Autodesk Fusion 360 part; units mm, degrees
sketch "Sketch2" plane through (0, 0, 0) normal (0, 0, 1) x (1, 0, 0)
  line L0 (0, 0) -> (2, 0)
  line L1 (2, 0) -> (2, 10)
  line L2 (2, 10) -> (0, 10)
  line L3 (0, 10) -> (0, 0)
  line L4 (0, 10) -> (2, 10)
  line L5 (2, 10) -> (2, 12)
  line L6 (2, 12) -> (0, 12)
  line L7 (0, 12) -> (0, 10)
  line L8 (0, 10) -> (-5, 10)
  line L9 (-5, 10) -> (-5, 12)
  line L10 (-5, 12) -> (0, 12)
  line L11 (0, 12) -> (0, 10)
  line L12 (-5, 10) -> (-7, 10)
  line L13 (-7, 10) -> (-7, 12)
  line L14 (-7, 12) -> (-5, 12)
  line L15 (-5, 12) -> (-5, 10)
  line L16 (-7, 10) -> (-5, 10)
  line L17 (-5, 10) -> (-5, -14)
  line L18 (-5, -14) -> (-7, -14)
  line L19 (-7, -14) -> (-7, 10)
  line L20 (-7, -14) -> (-5, -14)
  line L21 (-5, -14) -> (-5, -16)
  line L22 (-5, -16) -> (-7, -16)
  line L23 (-7, -16) -> (-7, -14)
  line L24 (-7, -16) -> (-30, -16)
  line L25 (-30, -16) -> (-30, -14)
  line L26 (-30, -14) -> (-7, -14)
  line L27 (-7, -14) -> (-7, -16)
  line L28 (-30, -16) -> (-32, -16)
  line L29 (-32, -16) -> (-32, -14)
  line L30 (-32, -14) -> (-30, -14)
  line L31 (-30, -14) -> (-30, -16)
  line L32 (-32, -14) -> (-30, -14)
  line L33 (-30, -14) -> (-30, 10)
  line L34 (-30, 10) -> (-32, 10)
  line L35 (-32, 10) -> (-32, -14)
  dimension "d3" = 2
  dimension "d4" = 10
  dimension "d5" = 2
  dimension "d6" = 2
  dimension "d7" = 5
  dimension "d8" = 2
  dimension "d9" = 2
  dimension "d10" = 2
  dimension "d11" = 24
  dimension "d12" = 2
  dimension "d13" = 23
  dimension "d14" = 2
  dimension "d15" = 2
  dimension "d16" = 2
  dimension "d17" = 2
  dimension "d18" = 24
extrude "Extrude1" add sketch "Sketch2" along normal blind 36
sketch "Sketch3" plane through (0, -16, 0) normal (0, -1, 0) x (1, 0, 0)
  line L0 (-32, 0) -> (-5, 0)
  line L1 (-5, 0) -> (-5, 36)
  line L2 (-5, 36) -> (-32, 36)
  line L3 (-32, 36) -> (-32, 0)
  line L4 (-5, 18) -> (-7, 18) construction
  line L5 (-7, 18) -> (-10.5, 18) construction
  line L6 (-14, 12) -> (-7, 12)
  line L7 (-7, 12) -> (-7, 24)
  line L8 (-7, 24) -> (-14, 24)
  line L9 (-14, 24) -> (-14, 12)
  line L10 (-14, 12) -> (-7, 24) construction
  line L11 (-7, 12) -> (-14, 24) construction
  point P0 (-7, 18)
  point P1 (-10.5, 18)
  dimension "d23" = 2
  dimension "d28" = 3.5
  dimension "d29" = 7
  dimension "d30" = 12
extrude "Extrude3" cut sketch "Sketch3" against normal blind 3 contours L6 L7 L8 L9
fillet "Fillet1" radius 0.5 8 edges at (0, 0, 18) (2, 0, 18) (-5, -16, 18) (-32, -16, 18) (2, 12, 18) (-7, 12, 18) (-30, 10, 18) (-32, 10, 18)
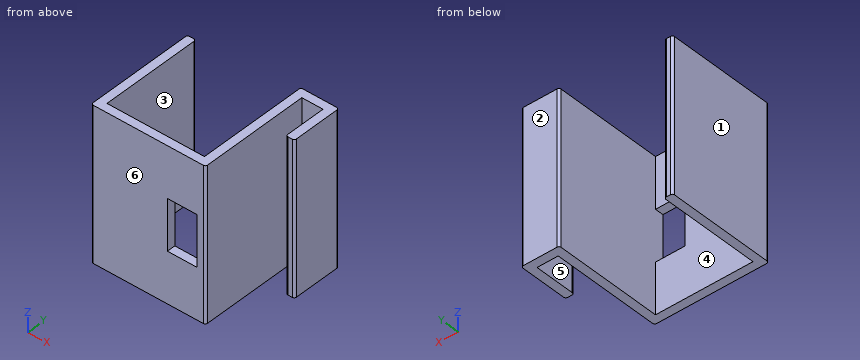
Verification items for the finished model (mm, model axes). Face numbers are marked on the shaded views. A direction names the side the tool comes from. Give positions to 0.01 mm unless a question says otherwise; leave off trailing zeros. Loops run counter-clockwise (first coordinate to the right, second up) from the corner with the lowest first, then second, coordinate; pieces in that order, holes last.
1. Mould release check, pull along X, two halves, no side actions. Record for the marked faces 1, 2 and 3: released by +X, released by -X, zero draft, split by the parting line, or undercut.
2. Set-up check for the marked faces 4, 5 and 6: record each of +Z, -Z, +X, -X, +Y, -Y from which the full face is reachable in a straight line by a thin tool's end or side.
3. Section check D-D, the plane x = -12.5. Enter the section's corners in (y, z), then the cut area to 3 significant figures.
4. Section check B-B, the plane y = -8.25. Enter the section's corners in (x, z), then the cut area to 3 significant figures.
5. Thickness scan on line 1 (X direction, y = 4.75, z = 20.5); line 2 (X direction, y = -8, z = 30.5); line 3 (X direction, y = -14.5, z = 14). Record the ranges inside material, lowest first.
6. Section check A-A, the plane y = 9. Enter the section's corners in (x, z).
7. Go/stop test with flat-tipped pins: pin 1 Ø1.1 at (x, z) = (1, 12.5) entering from -Y; pin 2 Ø0.6 at (y, z) = (-15, 20) entering from +X; pin 3 Ø5 at (x, z) = (-18, 23) entering from +Y; pin 4 Ø6 at (x, y) = (-19, -10) entering from +Z. Record where each tip stops, or that it passes through.
8. Section check C-C, the plane z = 13. Enter the section's corners in (x, y).
Geometry says:
1. face 1: released by -X
1. face 2: zero draft
1. face 3: undercut
2. face 4: +Z, -Z, +Y
2. face 5: +Z, -Z, -Y
2. face 6: +Z, -Z, +X, -X, -Y
3. outline: (-16, 0) - (-14, 0) - (-14, 12) - (-16, 12) - close; (-16, 24) - (-14, 24) - (-14, 36) - (-16, 36) - close
3. area: 48.0 mm2
4. outline: (-32, 0) - (-30, 0) - (-30, 36) - (-32, 36) - close; (-7, 0) - (-5, 0) - (-5, 36) - (-7, 36) - close
4. area: 144 mm2
5. line 1: x = -32 to -30, -7 to -5, 0 to 2
5. line 2: x = -32 to -30, -7 to -5
5. line 3: x = -32 to -14, -7 to -5
6. outline: (-32, 0) - (-30, 0) - (-30, 36) - (-32, 36) - close; (-7, 0) - (-5, 0) - (-5, 36) - (-7, 36) - close; (0, 0) - (2, 0) - (2, 36) - (0, 36) - close
7. pin 1: stops at y = 0
7. pin 2: stops at x = -5
7. pin 3: stops at y = -14
7. pin 4: passes through
8. outline: (-32, -15.5) arc R0.5 ccw to (-31.5, -16) - (-14, -16) - (-14, -14) - (-30, -14) - (-30, 9.5) arc R0.5 ccw to (-30.5, 10) - (-31.5, 10) arc R0.5 ccw to (-32, 9.5) - close; (-7, -16) - (-5.5, -16) arc R0.5 ccw to (-5, -15.5) - (-5, 10) - (0, 10) - (0, 0.5) arc R0.5 ccw to (0.5, 0) - (1.5, 0) arc R0.5 ccw to (2, 0.5) - (2, 11.5) arc R0.5 ccw to (1.5, 12) - (-6.5, 12) arc R0.5 ccw to (-7, 11.5) - close
